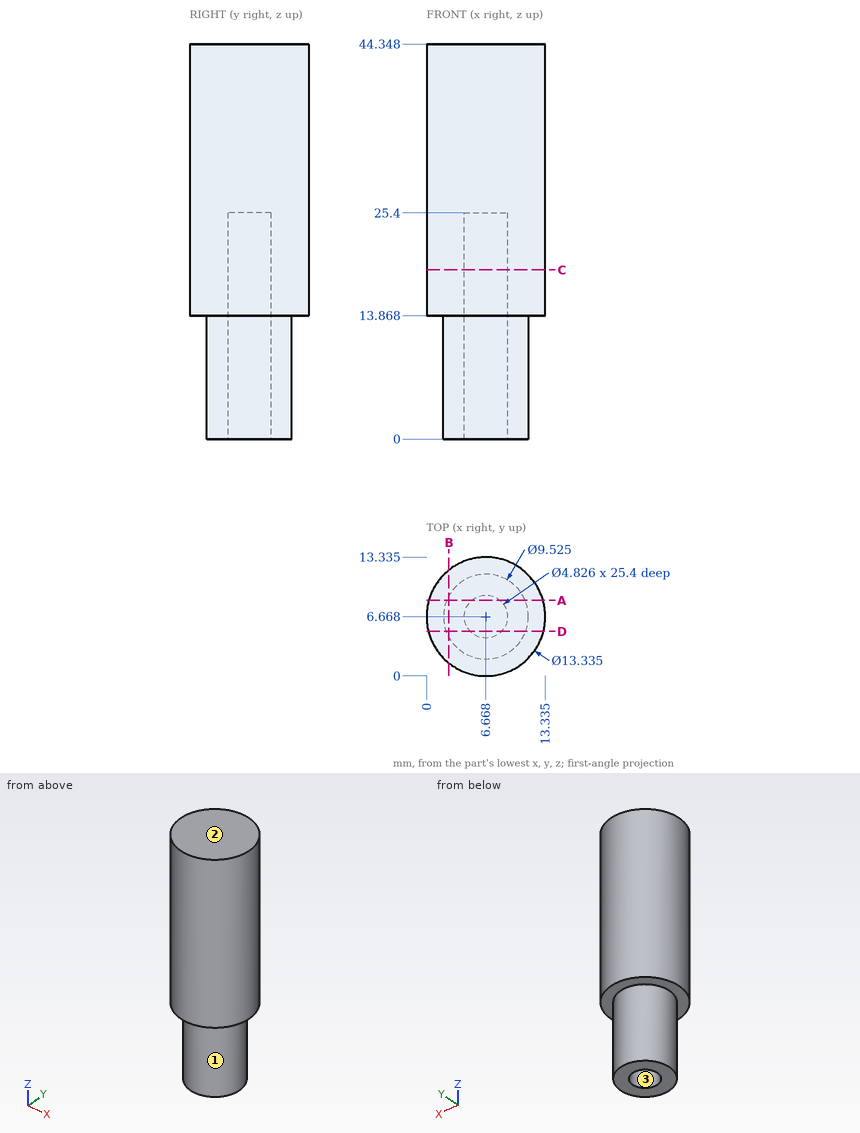
Design review of the part shown in the three views and the two pictorial views. Dimensions are in mm from the part's minimum x, y and z. Round coordinates to 2 decimals unless told otherwise and drop trailing zeros. Loops run counter-clockwise (first coordinate to the right, second up) from the corner with the lowest first, then second, coordinate; pieces in that order, holes last.
(1) We need section C-C (z = 19). Give the boundary of the cut face in (x, y) (1 decimal), plus the area to 3 significant figures.
Returned:
outline: circle Ø13.3 at (6.7, 6.7); hole circle Ø4.8 at (6.7, 6.7)
area: 121 mm2
(2) We need section D-D (y = 5). Give the boundary of the cut face in (x, z).
Returned:
outline: (0.21, 13.87) - (2.21, 13.87) - (2.21, 0) - (4.92, 0) - (4.92, 25.4) - (8.41, 25.4) - (8.41, 0) - (11.13, 0) - (11.13, 13.87) - (13.12, 13.87) - (13.12, 44.35) - (0.21, 44.35) - close
(3) We need section A-A (y = 8.5). Give the boundary of the cut face in (x, z), plus the area to 3 significant figures.
Returned:
outline: (0.26, 13.87) - (2.27, 13.87) - (2.27, 0) - (5.1, 0) - (5.1, 25.4) - (8.24, 25.4) - (8.24, 0) - (11.06, 0) - (11.06, 13.87) - (13.08, 13.87) - (13.08, 44.35) - (0.26, 44.35) - close
area: 433 mm2
(4) Clearance check with flat-ended pins moving along their axes: P1, Ø8, axis at x = 1.5, z = 24, coming from the -Y side; P2, Ø1, axis at y = 6, z = 32.5, coming from the +X side; P3, Ø2, axis at x = 12, y = 2.5, coming from the -Z side. State where each tip first meets the part, or that it passes through.
Returned:
P1: stops at y = 0.1
P2: stops at x = 13.33
P3: stops at z = 13.87
(5) We need section B-B (x = 2.5). Give the boundary of the cut face in (y, z).
Returned:
outline: (1.46, 13.87) - (4.36, 13.87) - (4.36, 0) - (8.97, 0) - (8.97, 13.87) - (11.87, 13.87) - (11.87, 44.35) - (1.46, 44.35) - close
(6) Mouldability with a two-part tool opening along Y and no side actions: class the marked faces 1, 2 and 3 as released by +Y, released by -Y, zero draft, split by the parting line, or undercut.
Returned:
face 1: split by the parting line
face 2: zero draft
face 3: undercut
(7) Wall thickness on line 1 along Z through (x, y) = (2.25, 4.5); line 2 along Z through (x, y) = (7.25, 6.5); line 3 along X through (y, z) = (9.75, 37) (1 decimal): over which ranges is each line inside the solid? List them lowest first.
Returned:
line 1: z = 13.87 to 44.35
line 2: z = 25.4 to 44.35
line 3: x = 0.8 to 12.6
